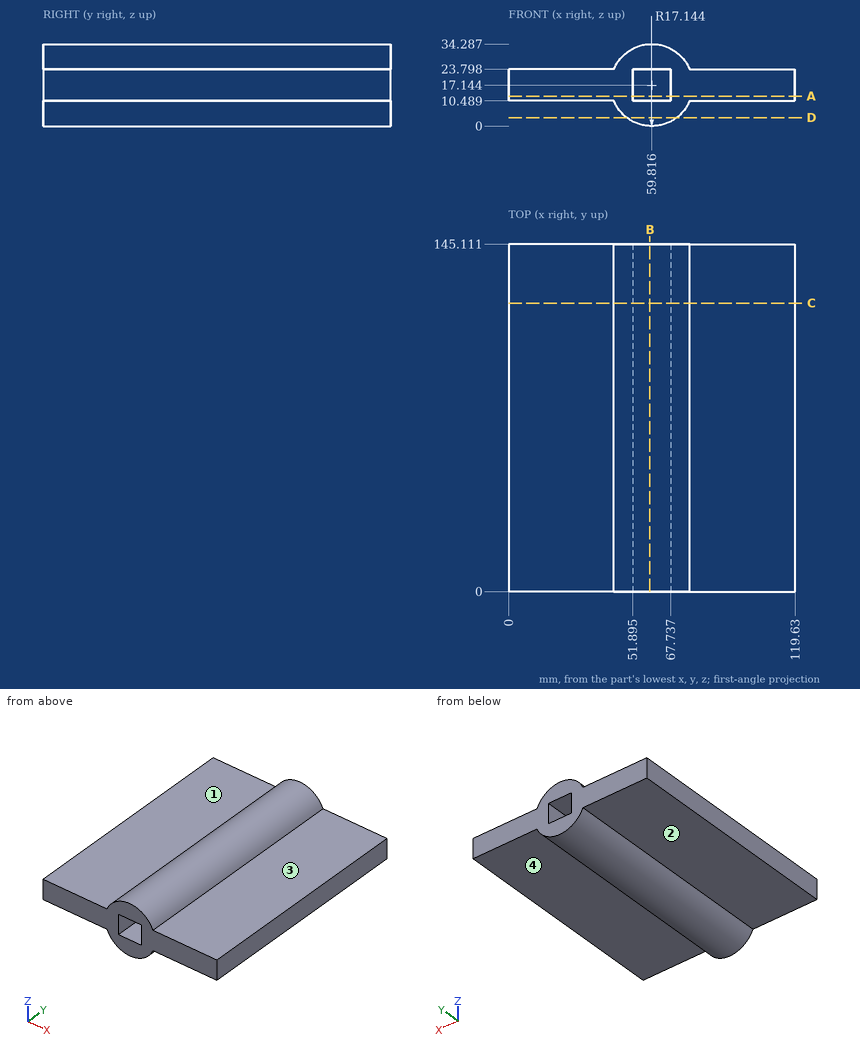
Job drawing, mm, ordinate dimensions from the low corner. One solid piece. A direction names the side the tool comes from. Coordinates: 2 decimals unless noted, no trailing zeros. Order: outer loops, then holes, each group sorted by start corner. A loop starts at its lowest first (then second) coordinate and runs counter-clockwise, first axis right, second up. Notation, with made-up numbers: (9.5, 40.5) -> (66.5, 40.5) arc R15 ccw to (66.5, 56.5) -> close; hole circle Ø9 at (-26.5, -3.75). An arc over 180 degrees is marked (long way). Return JSON: item names as keys, results as strings. Group by question number.
Item 1: Saw through at A-A on z = 12.5. Write the cut outline in (x, y) (1 decimal), then the cut area to 3 significant figures.
Item 2: Saw through at C-C on y = 120.5. Write the cut outline in (x, z) (1 decimal), then the cut area to 3 significant figures.
Item 3: Tool access for the marked faces 1, 2, 3 and 4: list every direction of +Z, -Z, +X, -X, +Y, -Y with a clear straight run to the whole face (end or side of a thin tool).
Item 4: Saw through at D-D on z = 3.5. Write the cut outline in (x, y) (1 decimal).
Item 5: Saw through at B-B on x = 59. Write the cut outline in (y, z).
Item 6: Flat gauge pins, fed straight in: P1, Ø5, axis at y = 128.5, z = 29.5, coming from the -X side; P2, Ø12, axis at y = 18.5, z = 3.5, coming from the +X side; P3, Ø6, axis at x = 97.5, y = 116.5, coming from the -Z side. Where does each tip first touch, or does it go through?
Item 7: Wall check: line 1 along X through (y, z) = (109, 17.5) (1 decimal); line 2 along Z through (x, y) = (82.5, 50); line 3 along Z through (x, y) = (66.5, 31.5) (1 decimal). Give the ranges that are in metal, low to high. Write a range as [from, to].
Values found:
{
 "1": {"outline": "(0, 0) -> (51.9, 0) -> (51.9, 145.1) -> (0, 145.1) -> close; (67.7, 0) -> (119.6, 0) -> (119.6, 145.1) -> (67.7, 145.1) -> close", "area": "15,100 mm2"},
 "2": {"outline": "(0, 10.5) -> (44, 10.5) arc R17.1 ccw to (75.6, 10.5) -> (119.6, 10.5) -> (119.6, 23.8) -> (75.6, 23.8) arc R17.1 ccw to (44, 23.8) -> (0, 23.8) -> close; hole (51.9, 10.5) -> (67.7, 10.5) -> (67.7, 23.8) -> (51.9, 23.8) -> close", "area": "1,860 mm2"},
 "3": {"face 1": "+Z, -X, +Y, -Y", "face 2": "-Z, -X, +Y, -Y", "face 3": "+Z, +X, +Y, -Y", "face 4": "-Z, +X, +Y, -Y"},
 "4": {"outline": "(49.4, 0) -> (70.2, 0) -> (70.2, 145.1) -> (49.4, 145.1) -> close"},
 "5": {"outline": "(0, 0.02) -> (145.11, 0.02) -> (145.11, 10.49) -> (0, 10.49) -> close; (0, 23.8) -> (145.11, 23.8) -> (145.11, 34.27) -> (0, 34.27) -> close"},
 "6": {"P1": "stops at x = 45.79", "P2": "stops at x = 75.16", "P3": "stops at z = 10.49"},
 "7": {"line 1": "x = [0, 51.9], [67.7, 119.6]", "line 2": "z = [10.49, 23.8]", "line 3": "z = [1.4, 10.5], [23.8, 32.9]"}
}
